For this review, take the finished solid that the model builds, in its own axes (mm). Face numbers are marked on the shaded views. A direction names the side the tool comes from. Coordinates: 2 decimals unless noted, no trailing zeros. Order: outer loops, then holes, each group sorted by start corner. A loop starts at its lowest first (then second) coordinate and runs counter-clockwise, first axis right, second up. Notation, with made-up numbers: (67, -39) - (114, -39) arc R23 cw to (114, -7) - close; hole circle Ø8 at (-11.75, 41). An arc over 180 degrees is marked (long way). One line per item, written item: value. Start each with the question number.
(1) Consider section C-C on y = 3. Write out the cut boundary in (x, z), then the cut area to 3 significant figures.
(2) Clearance check with flat-ended pins moving along their axes: pin 1 (1 mm diameter, centred on y = 7.5, z = -5, fed in from +X); pin 2 (6 mm diameter, centred on x = 46.5, z = -2, fed in from -Y); pin 3 (2.5 mm diameter, centred on x = 18.5, y = 6.5, fed in from -Z). State where each tip first meets the part, or that it passes through.
(3) For the marked faces 4, 5 and 6, list the 3-axis set-ups (+Z, -Z, +X, -X, +Y, -Y) from which the entire face can be reached by the end or side of a thin tool; tool diameter is ignored.
(4) Consider section B-B on z = 0. Write out the cut boundary in (x, y).
(5) Mouldability with a two-part tool opening along X and no side actions: class the marked faces 1, 2 and 3 as released by +X, released by -X, zero draft, split by the parting line, or undercut.
(6) Consider section D-D on z = 7.25. Write out the cut boundary in (x, y).
(7) To check wall thickness, follow line 1 along Z through (x, y) = (60, 3.25); line 2 along X through (y, z) = (4, -3.5); line 3 along Z through (x, y) = (3, 1). State the ranges of each line that lie inside material, in increasing order.
(8) Consider section A-A on x = 0. Write out the cut boundary in (y, z).
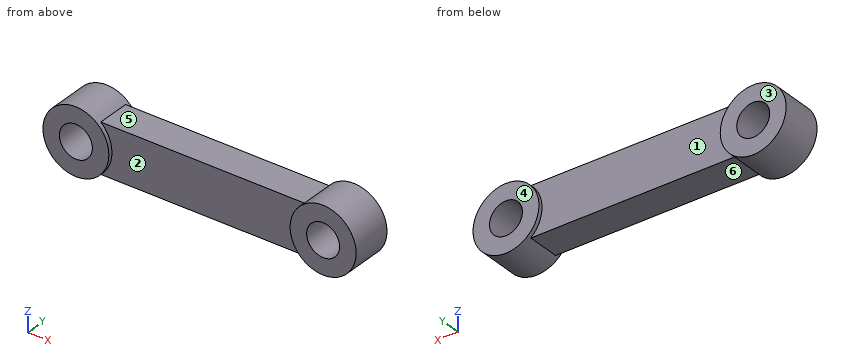
```python
from build123d import *

# Parameters (mm, degrees)
SKETCH_1_R        = 8
SKETCH_1_R_2      = 4
EXTRUDE_1_DEPTH   = 10
EXTRUDE_1_2_DEPTH = 10
EXTRUDE_START     = 1
EXTRUDE_2_DEPTH   = 8


with BuildPart() as part:
    # Sketch 1 → Extrude 1 (new body)
    with BuildSketch(Plane(origin=(0, 0, 0), x_dir=(1, 0, 0), z_dir=(0, 1, 0))):
        Circle(SKETCH_1_R)
        Circle(SKETCH_1_R_2, mode=Mode.SUBTRACT)
    extrude(amount=EXTRUDE_1_DEPTH)



with BuildPart() as body_2:
    # Sketch 1 → Extrude 1 2 (new body)
    with BuildSketch(Plane(origin=(0, 0, 0), x_dir=(1, 0, 0), z_dir=(0, 1, 0))):
        with Locations((60, 0)):
            Circle(SKETCH_1_R)
        with Locations((60, 0)):
            Circle(SKETCH_1_R_2, mode=Mode.SUBTRACT)
    extrude(amount=EXTRUDE_1_2_DEPTH)


with BuildPart() as part_1:
    add(part.part)

    add(body_2.part)  # Extrude 2 merges body 2
    # Sketch 2 → Extrude 2 (add)
    with BuildSketch(Plane(origin=(0, 0, 0), x_dir=(1, 0, 0), z_dir=(0, 1, 0)).offset(EXTRUDE_START)):
        with BuildLine():
            Line((5.291502622, -6), (54.708497378, -6))
            ThreePointArc((54.708497378, -6), (52, 0), (54.708497378, 6))
            Line((54.708497378, 6), (5.291502622, 6))
            ThreePointArc((5.291502622, 6), (8, 0), (5.291502622, -6))
        make_face()
    extrude(amount=EXTRUDE_2_DEPTH)


solid = part_1.part
```
Geometry check:
1. outline: (5.29, -6) - (54.71, -6) arc R8 ccw (long way) to (54.71, 6) - (5.29, 6) arc R8 ccw (long way) to start; hole circle Ø8 at (0, 0); hole circle Ø8 at (60, 0)
1. area: 850 mm^2
2. pin 1: stops at x = 66.61
2. pin 2: stops at y = 1
2. pin 3: stops at z = -6
3. face 4: +Z, -Z, +X, -X, +Y
3. face 5: +Z, +Y, -Y
3. face 6: -Z, +Y, -Y
4. outline: (-8, 0) - (-4, 0) - (-4, 10) - (-8, 10) - close; (4, 0) - (8, 0) - (8, 1) - (52, 1) - (52, 0) - (56, 0) - (56, 10) - (52, 10) - (52, 9) - (8, 9) - (8, 10) - (4, 10) - close; (64, 0) - (68, 0) - (68, 10) - (64, 10) - close
5. face 1: undercut
5. face 2: undercut
5. face 3: zero draft
6. outline: (-3.38, 0) - (3.38, 0) - (3.38, 10) - (-3.38, 10) - close; (56.62, 0) - (63.38, 0) - (63.38, 10) - (56.62, 10) - close
7. line 1: z = -8 to -4, 4 to 8
7. line 2: x = -7.19 to -1.94, 1.94 to 58.06, 61.94 to 67.19
7. line 3: z = -7.42 to -2.65, 2.65 to 7.42
8. outline: (0, -8) - (10, -8) - (10, -4) - (0, -4) - close; (0, 4) - (10, 4) - (10, 8) - (0, 8) - close
